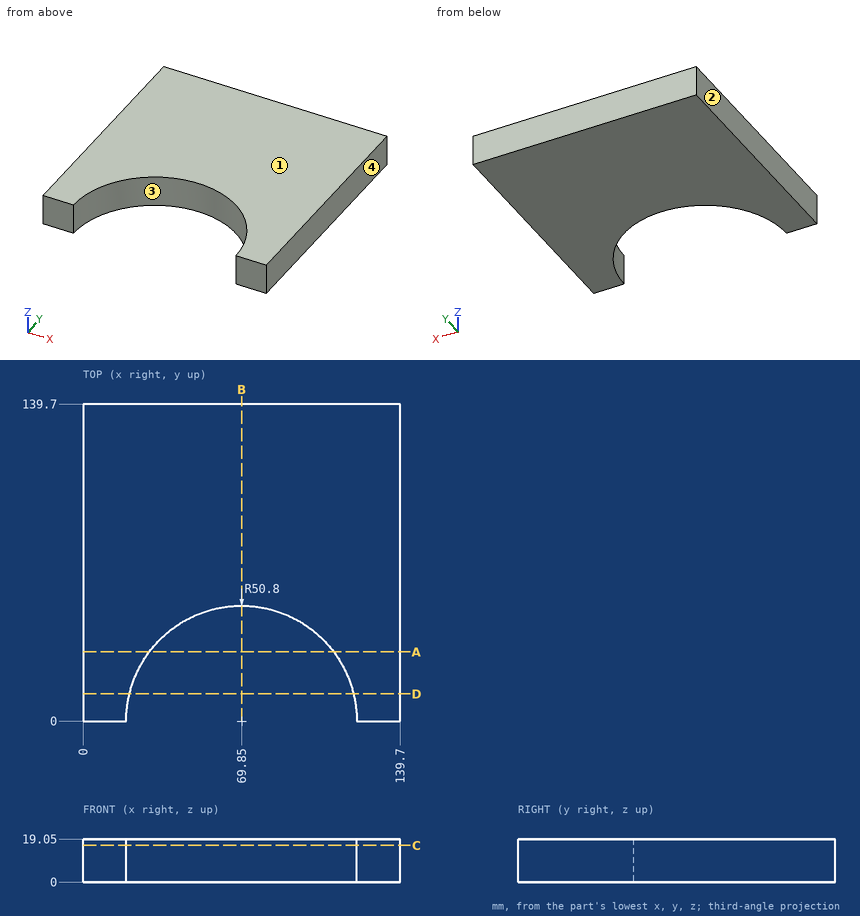
Drawing for the job (mm, zero at the part's lowest x, y, z). Round coordinates to 2 decimals unless told otherwise and drop trailing zeros. Write each loop counter-clockwise with the first axis right and the second up, starting at its lowest first coordinate (ties: lowest second). Pieces come first, ordered by that corner, then holes. Notation, with made-up numbers: (13.25, 81) - (67.25, 81) arc R30 ccw to (67.25, 103) - close; hole circle Ø5 at (40, 66.25). An arc over 180 degrees is marked (long way). Use CSV: the item, a comma, the result in double quotes.
(1) Band-saw the part on A-A (y = 30.5). Write the cut outline in (x, z) (3 decimals).
Response:
outline,"(0, 0) - (29.225, 0) - (29.225, 19.05) - (0, 19.05) - close; (110.475, 0) - (139.7, 0) - (139.7, 19.05) - (110.475, 19.05) - close"
(2) Wall check: line 1 (X direction, y = 43, z = 14); line 2 (X direction, y = 21, z = 10.5); line 3 (Y direction, x = 51.5, z = 2.75). Give the ranges that are in metal, low to high.
Response:
line 1,"0 to 42.8, 96.9 to 139.7"
line 2,"0 to 23.59, 116.11 to 139.7"
line 3,"47.37 to 139.7"
(3) Mould opens along X. For the marked faces 1, 2, 3 and 4 say: pulls with the +X half, pulls with the -X half, needs draft (parallel to the pull), parting line crosses it, or undercut.
Response:
face 1,"needs draft"
face 2,"pulls with the -X half"
face 3,"undercut"
face 4,"pulls with the +X half"
(4) Band-saw the part on B-B (x = 69.85). Write the cut outline in (y, z).
Response:
outline,"(50.8, 0) - (139.7, 0) - (139.7, 19.05) - (50.8, 19.05) - close"
(5) Band-saw the part on C-C (z = 16.25). Write the cut outline in (x, y), plus the area to 3 significant figures.
Response:
outline,"(0, 0) - (19.05, 0) arc R50.8 cw to (120.65, 0) - (139.7, 0) - (139.7, 139.7) - (0, 139.7) - close"
area,"15,500 mm²"
(6) Band-saw the part on D-D (y = 12). Write the cut outline in (x, z), plus the area to 3 significant figures.
Response:
outline,"(0, 0) - (20.49, 0) - (20.49, 19.05) - (0, 19.05) - close; (119.21, 0) - (139.7, 0) - (139.7, 19.05) - (119.21, 19.05) - close"
area,"781 mm²"
